Geometry: see drawing. Coordinates: mm, zero at the bounding-box minimum. Round coordinates to 2 decimals unless told otherwise and drop trailing zeros. Loops run counter-clockwise (first coordinate to the right, second up) from the corner with the lowest first, then second, coordinate; pieces in that order, holes last.
(1) First-contact query: pin 1 Ø3 at (x, y) = (42, 241.5) entering from +Z. Flat tip, straight axial feed; report the tip coordinate or a pass-through.
(2) Section A-A, the plane y = 175. Return the cut outline in (x, z), plus the area to 3 significant figures.
(3) Material intervals for probe 1 along Z at (x, y) = (16.5, 52), sorted ascending.
(4) Section B-B, the plane z = 7.25. Return the cut outline in (x, y).
(5) Section D-D, the plane x = 20. Return the cut outline in (y, z).
(6) Section C-C, the plane x = 150. Return the cut outline in (y, z).
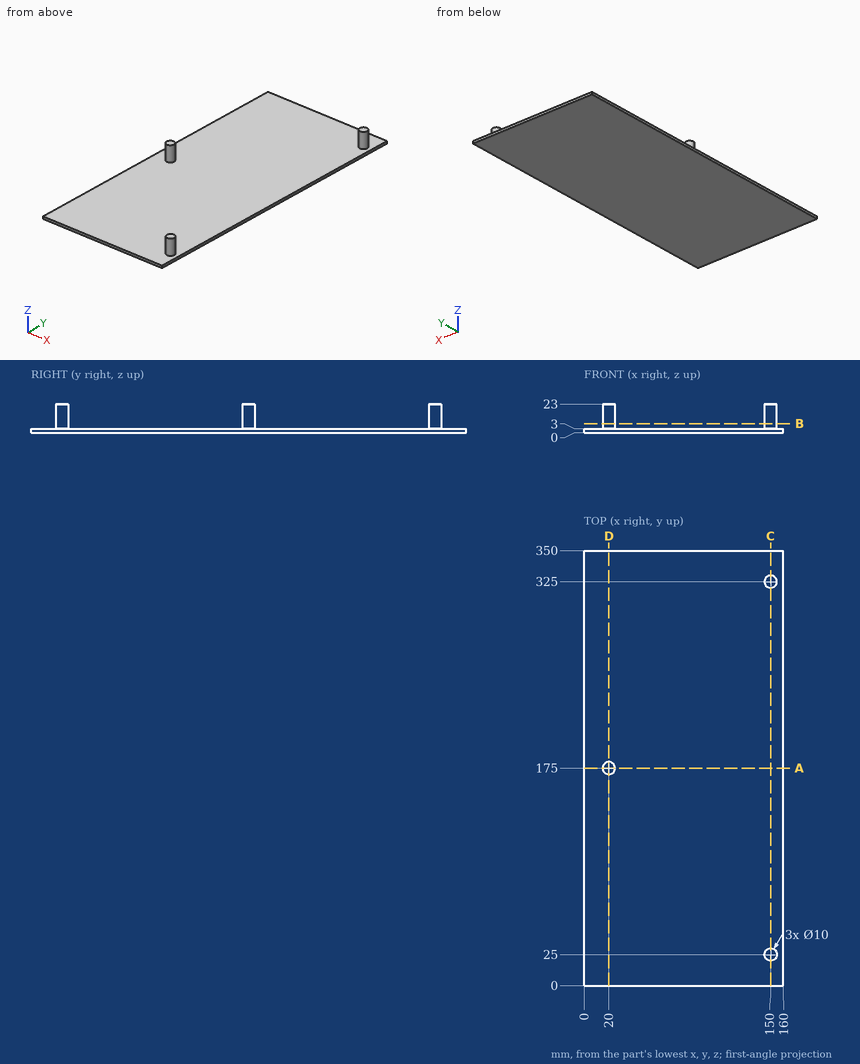
Output values:
1. pin 1: stops at z = 3
2. outline: (0, 0) - (160, 0) - (160, 3) - (25, 3) - (25, 23) - (15, 23) - (15, 3) - (0, 3) - close
2. area: 680 mm2
3. probe 1: z = 0 to 3
4. outline: circle Ø10 at (20, 175); circle Ø10 at (150, 25); circle Ø10 at (150, 325)
5. outline: (0, 0) - (350, 0) - (350, 3) - (180, 3) - (180, 23) - (170, 23) - (170, 3) - (0, 3) - close
6. outline: (0, 0) - (350, 0) - (350, 3) - (330, 3) - (330, 23) - (320, 23) - (320, 3) - (30, 3) - (30, 23) - (20, 23) - (20, 3) - (0, 3) - close
